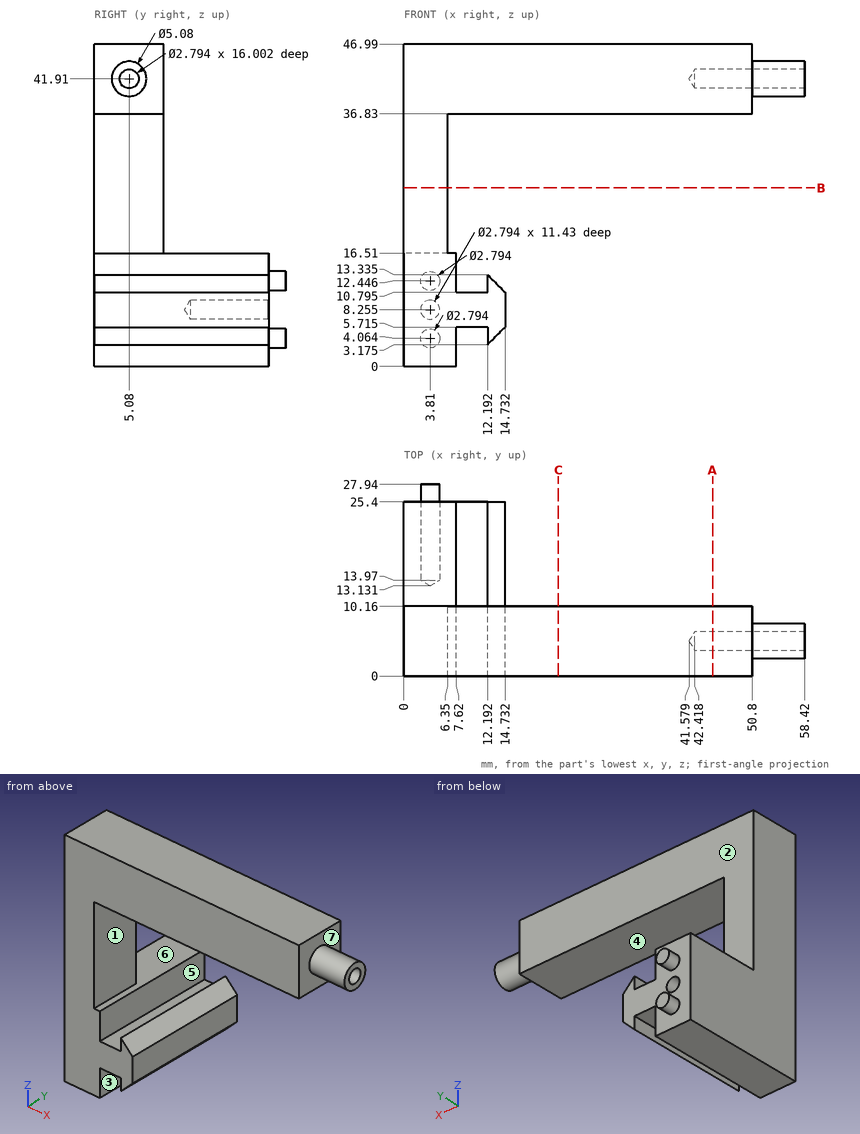
Input: dimensioned drawing with shaded views. Units: mm. Origin: part minimum x, y, z. A direction names the side the tool comes from. Give positions to 0.01 mm unless a question says otherwise; leave off trailing zeros. Write each loop counter-clockwise with the first axis right and the second up, starting at its lowest first coordinate (ties: lowest second). Pieces come first, ordered by that corner, then holes. Notation, with made-up numbers: (-27.75, -21) - (-8.75, -21) arc R28 cw to (-8.75, 13) - close; hole circle Ø3 at (44, -25.75). An arc over 180 degrees is marked (long way). Write item = value, one per line. Start each with the question number.
1) Reachability of the marked faces 4, 5, 6 and 7 from +Z, -Z, +X, -X, +Y, -Y: full face, straight path, thin tool, end or side. Return the list, or none.
2) Cut plane B-B (z = 26). Return loops of the section in (x, y), and give its area (3 significant figures).
3) Material intervals for L1, parallel to Z at x = 49.25, y = 5.08; L2, parallel to Y at x = 54.75, z = 41.91; L3, parallel to Z at x = 7, y = 3, sorted ascending. Write a range as [from, to].
4) Draft query along X for the marked faces 1, 2 and 3. Return one class per face: pulls with the +X half, pulls with the -X half, needs draft (parallel to the pull), parting line crosses it, or undercut.
5) Cut plane A-A (x = 45). Return loops of the section in (y, z).
6) Cut plane C-C (x = 22.5). Return loops of the section in (y, z).
7) Pin query (flat end, axial travel): pin 1 (3 mm diameter, centred on y = 7, z = 27, fed in from +X); pin 2 (8 mm diameter, centred on x = 32.5, y = 3.5, fed in from -Z); pin 3 (1.7 mm diameter, centred on y = 5.08, z = 41.91, fed in from +X). Return the tip coordinate at first contact, or that it passes through.
Answers follow:
q1.face_4 = +X, +Y, -Y
q1.face_5 = +Y, -Y
q1.face_6 = +X, +Y
q1.face_7 = +X
q2.outline = (0, 0) - (6.35, 0) - (6.35, 10.16) - (0, 10.16) - close
q2.area = 64.5 mm^2
q3.L1 = [36.83, 40.51], [43.31, 46.99]
q3.L2 = [2.54, 3.68], [6.48, 7.62]
q3.L3 = [0, 16.51], [36.83, 46.99]
q4.face_1 = pulls with the +X half
q4.face_2 = needs draft
q4.face_3 = undercut
q5.outline = (0, 36.83) - (10.16, 36.83) - (10.16, 46.99) - (0, 46.99) - close; hole circle Ø2.79 at (5.08, 41.91)
q6.outline = (0, 36.83) - (10.16, 36.83) - (10.16, 46.99) - (0, 46.99) - close
q7.pin_1 = 6.35
q7.pin_2 = 36.83
q7.pin_3 = 42.09
